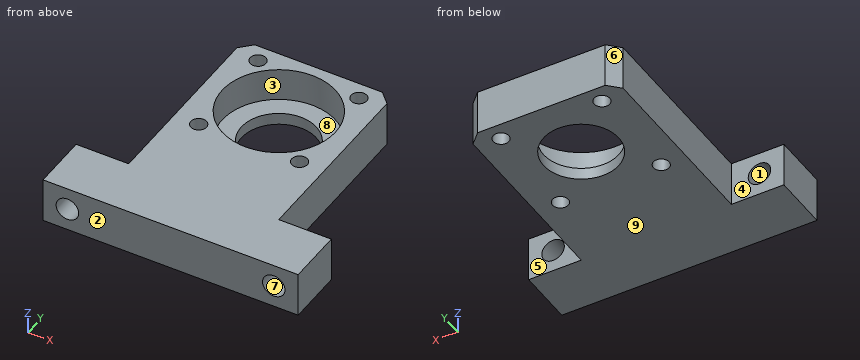
from build123d import *

# Parameters (mm, degrees)
SKETCH_1_W          = 68
SKETCH_1_H          = 67
EXTRUDE_1_DEPTH     = 12
SKETCH_2_R          = 15.1
CUT_EXTRUDE_1_DEPTH = 8.8
SKETCH_3_R          = 10
CUT_EXTRUDE_2_DEPTH = 96.866782568
HOLE_WIZARD_M5_1_D  = 4.2
SKETCH_7_W          = 14
SKETCH_7_H          = 52
CUT_EXTRUDE_3_DEPTH = 97.213304693
CHAMFER_1_SIZE      = 3
SKETCH_8_R          = 3
CUT_EXTRUDE_4_DEPTH = 97.213304693


with BuildPart() as part:
    # 草图1 → 凸台-拉伸1 (new body)
    with BuildSketch(Plane.XY):
        with Locations((34, 33.5)):
            Rectangle(SKETCH_1_W, SKETCH_1_H)
    extrude(amount=EXTRUDE_1_DEPTH)

    # 草图2 → 切除-拉伸1 (cut)
    with BuildSketch(Plane.XY.offset(12)):
        with Locations((34, 49)):
            Circle(SKETCH_2_R)
    extrude(amount=-CUT_EXTRUDE_1_DEPTH, mode=Mode.SUBTRACT)

    # 草图3 → 切除-拉伸2 (cut, through all)
    with BuildSketch(Plane.XY.offset(3.2)):
        with Locations((34, 49)):
            Circle(SKETCH_3_R)
    extrude(amount=-CUT_EXTRUDE_2_DEPTH, mode=Mode.SUBTRACT)

    # M5 螺纹孔1 (through all)
    with Locations(Plane.XY.offset(12)):
        with Locations((47.435028843, 62.435028843), (20.564971157, 62.435028843), (20.564971157, 35.564971157), (47.435028843, 35.564971157)):
            Hole(HOLE_WIZARD_M5_1_D / 2)

    # 草图7 → 切除-拉伸3 (cut, through all)
    with BuildSketch(Plane.XY.offset(12)):
        with Locations((7, 41)):
            Rectangle(SKETCH_7_W, SKETCH_7_H)
        with Locations((61, 41)):
            Rectangle(SKETCH_7_W, SKETCH_7_H)
    extrude(amount=-CUT_EXTRUDE_3_DEPTH, mode=Mode.SUBTRACT)

    # 倒角1
    chamfer_1_edges = [part.edges().sort_by_distance(p)[0] for p in [
        (14, 67, 6),
        (54, 67, 6),
    ]]
    chamfer(chamfer_1_edges, length=CHAMFER_1_SIZE)

    # 草图8 → 切除-拉伸4 (cut, through all)
    with BuildSketch(Plane.XZ):
        with Locations(Location((6.5, 6, 0), (0, 0, 270))):
            Circle(SKETCH_8_R)
        with Locations(Location((61.5, 6, 0), (0, 0, 270))):
            Circle(SKETCH_8_R)
    extrude(amount=-CUT_EXTRUDE_4_DEPTH, mode=Mode.SUBTRACT)


solid = part.part
Design review of the part built by this model. Coordinates are the model's own, in mm. Face numbers are marked on the shaded views. A direction names the side the tool comes from. Round coordinates to 2 decimals unless told otherwise and drop trailing zeros. Write each loop counter-clockwise with the first axis right and the second up, starting at its lowest first coordinate (ties: lowest second). Pieces come first, ordered by that corner, then holes. Notation, with made-up numbers: (53.25, 87) - (64.25, 87) arc R25 ccw to (64.25, 118) - close; hole circle Ø10 at (34.5, 16). An arc over 180 degrees is marked (long way). Return JSON: item names as keys, results as strings. Group by question number.
Item 1: Machinability: for the marked faces 1, 2, 3, 4 and 5, which of the approach directions +Z, -Z, +X, -X, +Y, -Y give a long, thin tool a straight path to every point of the face, cutting with its end or side? Answer none if there is none.
Item 2: For probe 1 along Y at (x, z) = (34, 8); probe 2 along Y at (x, z) = (22.5, 3.75); probe 3 along X at (y, z) = (62, 2), list the stretches that pass through material, from the lowest coordinate up. Write a range as [from, to].
Item 3: We need section C-C on y = 52. Write out the cut boundary in (x, z).
Item 4: We need section D-D on y = 8.5. Write out the cut boundary in (x, z).
Item 5: We need section B-B on x = 34. Write out the cut boundary in (y, z), and give its area (3 significant figures).
Item 6: The part is to be moulded in two halves that separate along Z. For the marked faces 6, 7, 8 and 9, say which applies: pulls with the +Z half, pulls with the -Z half, needs draft (parallel to the pull), parting line crosses it, or undercut.
Item 7: Insertion check: P1, Ø6.5, axis at x = 47.44, y = 62.44, coming from the +Z side; P2, Ø15, axis at x = 35, y = 42, coming from the +Z side; P3, Ø7, axis at x = 61.5, z = 6, coming from the +Y side; P4, Ø3.5, axis at y = 47.5, z = 5, coming from the +X side. Each pin has a flat end and moves straight along its axis. Give the tip position at first contact, or say it passes through.
Item 8: We need section A-A on z = 5.75. Write out the cut boundary in (x, y), and give its area (3 significant figures).
Model answer:
{
 "1": {"face 1": "+Y, -Y", "face 2": "+Z, -Z, +X, -X, -Y", "face 3": "+Z", "face 4": "+Z, -Z, -X, +Y", "face 5": "+Z, -Z, +X, +Y"},
 "2": {"probe 1": "y = [0, 33.9], [64.1, 67]", "probe 2": "y = [0, 34.75], [36.38, 39.21], [58.79, 61.62], [63.25, 67]", "probe 3": "x = [14, 18.51], [22.62, 45.38], [49.49, 54]"},
 "3": {"outline": "(14, 0) - (24.46, 0) - (24.46, 3.2) - (19.2, 3.2) - (19.2, 12) - (14, 12) - close; (43.54, 0) - (54, 0) - (54, 12) - (48.8, 12) - (48.8, 3.2) - (43.54, 3.2) - close"},
 "4": {"outline": "(0, 0) - (68, 0) - (68, 12) - (0, 12) - close; hole circle Ø6 at (6.5, 6); hole circle Ø6 at (61.5, 6)"},
 "5": {"outline": "(0, 0) - (39, 0) - (39, 3.2) - (33.9, 3.2) - (33.9, 12) - (0, 12) - close; (59, 0) - (67, 0) - (67, 12) - (64.1, 12) - (64.1, 3.2) - (59, 3.2) - close", "area": "474 mm²"},
 "6": {"face 6": "needs draft", "face 7": "undercut", "face 8": "pulls with the +Z half", "face 9": "pulls with the -Z half"},
 "7": {"P1": "stops at z = 12", "P2": "stops at z = 3.2", "P3": "stops at y = 15", "P4": "stops at x = 54"},
 "8": {"outline": "(0, 0) - (3.51, 0) - (3.51, 15) - (0, 15) - close; (9.49, 0) - (58.51, 0) - (58.51, 15) - (54, 15) - (54, 64) - (51, 67) - (17, 67) - (14, 64) - (14, 15) - (9.49, 15) - close; (64.49, 0) - (68, 0) - (68, 15) - (64.49, 15) - close; hole circle Ø4.2 at (20.56, 35.56); hole circle Ø4.2 at (20.56, 62.44); hole circle Ø30.2 at (34, 49); hole circle Ø4.2 at (47.44, 35.56); hole circle Ø4.2 at (47.44, 62.44)", "area": "2,140 mm²"}
}
